Here's how the part is built. I have some questions about the finished solid (model axes, mm). Give positions to 0.01 mm unless a question says otherwise; leave off trailing zeros. Write each loop counter-clockwise with the first axis right and the second up, starting at its lowest first coordinate (ties: lowest second). Pieces come first, ordered by that corner, then holes. Notation, with made-up numbers: M 3,20.5 L 32,20.5 A24 ccw 32,56.5 Z; hole C 63,-37 d9. An arc over 180 degrees is marked long. Answer as CSV lines item,"result". Start each with the question number.
Q1. If I drill on line 1 along X through (y, z) = (1, 0); line 2 along Z through (x, y) = (137.5, 1.3); line 3 along X through (y, z) = (1.4, 7.5), over which ranges is the centre line in solid material (lowest first)?
Q2. Suppose I cut it at A-A (x = 7). Write out the boundary of the cut face in (y, z), then the cut area to 3 significant figures.
Q3. Thinking about a two-plate mould opening in X: for faces 1 (the flat face through (66, 2, 0)), 2 (the cylindrical face through (-9.498, 0.986, 0.209)), 3 (the cylindrical face through (-8.464, 0.986, -0.325)), which applies, +X half, -X half, draft (parallel to the pull), parting line (faces both ways), or undercut?
Q4. Suppose I cut it at B-B (y = 0.35). Count the separate pieces of the cut face and the enclosed holes in it, then the cut area to 3 significant figures.
```python
from build123d import *

# Parameters (mm, degrees)
SKETCH_1_R      = 1.5
SKETCH_1_R_2    = 1
SKETCH_1_R_3    = 3
EXTRUDE_1_DEPTH = 2
FILLET_1_R      = 1


with BuildPart() as part:
    # Эскиз1 → Бобышка-Вытянуть1 (new body)
    with BuildSketch(Plane(origin=(0, 0, 0), x_dir=(1, 0, 0), z_dir=(0, 1, 0))):
        with BuildLine():
            Line((0, 9.5), (140, 9.5))
            Line((140, 9.5), (140, -9.5))
            Line((140, -9.5), (0, -9.5))
            ThreePointArc((0, -9.5), (-9.5, 0), (0, 9.5))
        make_face()
        with Locations(Location((0, 7, 0), (0, 0, 270))):
            Circle(SKETCH_1_R, mode=Mode.SUBTRACT)
        with Locations(Location((7, 0, 0), (0, 0, 270))):
            Circle(SKETCH_1_R, mode=Mode.SUBTRACT)
        with Locations(Location((0, -7, 0), (0, 0, 270))):
            Circle(SKETCH_1_R, mode=Mode.SUBTRACT)
        with Locations(Location((-7, 0, 0), (0, 0, 270))):
            Circle(SKETCH_1_R, mode=Mode.SUBTRACT)
        with Locations(Location((122.5, 7.5, 0), (0, 0, 270))):
            Circle(SKETCH_1_R_2, mode=Mode.SUBTRACT)
        with Locations(Location((137.5, 7.5, 0), (0, 0, 270))):
            Circle(SKETCH_1_R_2, mode=Mode.SUBTRACT)
        with Locations(Location((122.5, -7.5, 0), (0, 0, 270))):
            Circle(SKETCH_1_R_2, mode=Mode.SUBTRACT)
        with Locations(Location((137.5, -7.5, 0), (0, 0, 270))):
            Circle(SKETCH_1_R_2, mode=Mode.SUBTRACT)
        with Locations(Location((0, 0, 0), (0, 0, 270))):
            Circle(SKETCH_1_R_3, mode=Mode.SUBTRACT)
    extrude(amount=EXTRUDE_1_DEPTH)

    # Скругление1
    fillet_1_edges = [part.edges().sort_by_distance(p)[0] for p in [
        (140, 1, -9.5),
        (140, 1, 9.5),
    ]]
    fillet(fillet_1_edges, radius=FILLET_1_R)


solid = part.part
```
Resolved:
1,line 1,"-9.5 to -8.5, -5.5 to -3, 3 to 5.5, 8.5 to 140"
1,line 2,"-9.5 to -8.5, -6.5 to 6.5, 8.5 to 9.5"
1,line 3,"-5.83 to -1.41, 1.41 to 121.5, 123.5 to 136.5, 138.5 to 140"
2,outline,"M 0,-9.5 L 2,-9.5 L 2,-1.5 L 0,-1.5 Z; M 0,1.5 L 2,1.5 L 2,9.5 L 0,9.5 Z"
2,area,"32.0 mm^2"
3,face 1,"draft"
3,face 2,"-X half"
3,face 3,"undercut"
4,separate pieces,"1"
4,enclosed holes,"9"
4,area,"2,730 mm^2"
